from build123d import *

# Parameters (mm, degrees)
SKETCH1_R           = 6.5
BOSS_EXTRUDE1_DEPTH = 12
FILLET1_R           = 1


with BuildPart() as part:
    # Sketch1 → Boss-Extrude1 (new body)
    with BuildSketch(Plane.XY):
        with BuildLine():
            Line((-26, 9.287087811), (-26, 16.75))
            Line((-26, 16.75), (0, 16.75))
            Line((0, 16.75), (0, 20.75))
            Line((0, 20.75), (-30, 20.75))
            Line((-30, 20.75), (-30, 9.287087811))
            ThreePointArc((-30, 9.287087811), (-28, -9.5), (-26, 9.287087811))
        make_face()
        with Locations((-28, 0)):
            Circle(SKETCH1_R, mode=Mode.SUBTRACT)
    boss_extrude1 = extrude(amount=BOSS_EXTRUDE1_DEPTH)

    # Mirror1: Boss-Extrude1 across plane
    add(boss_extrude1.mirror(Plane(origin=(0, 0, 0), x_dir=(0, 0, 1), z_dir=(1, 0, 0))))

    # Fillet1
    fillet1_edges = [part.edges().sort_by_distance(p)[0] for p in [
        (-30, 9.287087811, 6),
        (-30, 20.75, 6),
        (-26, 16.75, 6),
        (-26, 9.287087811, 6),
        (26, 9.287087811, 6),
        (30, 9.287087811, 6),
        (30, 20.75, 6),
        (26, 16.75, 6),
    ]]
    fillet(fillet1_edges, radius=FILLET1_R)


solid = part.part
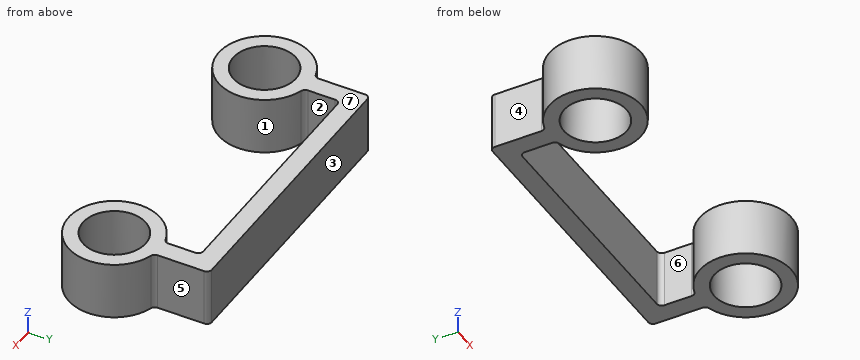
Can you work these out from the model? Positions are in its coordinate system, mm. Face numbers are marked on the shaded views. A direction names the side the tool comes from. Coordinates: 2 decimals unless noted, no trailing zeros. Order: outer loops, then holes, each group sorted by start corner. A loop starts at its lowest first (then second) coordinate and runs counter-clockwise, first axis right, second up. Notation, with made-up numbers: (33.5, -12.75) - (74.5, -12.75) arc R28 ccw to (74.5, 7.25) - close; hole circle Ø10 at (26.25, 41). An arc over 180 degrees is marked (long way). Answer as a JSON object with one key per item and string values. Group by question number.
Q1. Imagine slicing it at B-B (z = 1.5). Please give me the cut outline in (x, y), and give its area (3 significant figures).
Q2. On a 3-axis mill with a long thin cutter (end or side, diameter ignored), from which of +Z, -Z, +X, -X, +Y, -Y can I reach the whole of each face in a straight line? I mean the marked faces 5, 6 and 7. Say none if no direction works.
Q3. Imagine slicing it at A-A (x = -28). Please give me the cut outline in (y, z).
Q4. We'd pull the mould along X, two halves only. Please class the marked faces 1, 2, 3 and 4: +X half, -X half, draft (parallel to the pull), parting line (faces both ways), or undercut.
Q5. I need wall thicknesses on line 1 (Y direction, x = 28, z = 8); line 2 (X direction, y = 13, z = 5.25); line 3 (X direction, y = -4, z = 6). Which ranges of each line are inside material? Lowest first, please. Write a range as from..to.
Q6. Imagine slicing it at C-C (y = 0). Please give me the cut outline in (x, z).
Q7. Imagine slicing it at D-D (y = 19). Please give me the cut outline in (x, z).
Q8. Will these pins go through, and if not, where does the flat tip stop? P1, Ø3, axis at y = 11, z = 1.5, coming from the +X side; P2, Ø3, axis at y = 13, z = 6, coming from the +X side; P3, Ø10.5, axis at x = 28, y = 0, coming from the -Z side; P4, Ø1.7, axis at y = 12.5, z = 5, coming from the -X side.
Determined:
{
 "1": {"outline": "(-30.71, 9.1) arc R9.5 ccw (long way) to (-25.29, 9.1) arc R1 cw to (-26, 10.06) - (-26, 15.75) arc R1 cw to (-25, 16.75) - (25, 16.75) arc R1 cw to (26, 15.75) - (26, 10.06) arc R1 cw to (25.29, 9.1) arc R9.5 ccw (long way) to (30.71, 9.1) arc R1 cw to (30, 10.06) - (30, 19.75) arc R1 ccw to (29, 20.75) - (-29, 20.75) arc R1 ccw to (-30, 19.75) - (-30, 10.06) arc R1 cw to start; hole circle Ø13 at (-28, 0); hole circle Ø13 at (28, 0)", "area": "601 mm2"},
 "2": {"face 5": "+Z, -Z, +X, +Y", "face 6": "+Z, -Z", "face 7": "+Z, +X, -X, +Y, -Y"},
 "3": {"outline": "(-9.5, 0) - (-6.5, 0) - (-6.5, 12) - (-9.5, 12) - close; (6.5, 0) - (20.75, 0) - (20.75, 12) - (6.5, 12) - close"},
 "4": {"face 1": "undercut", "face 2": "undercut", "face 3": "draft", "face 4": "-X half"},
 "5": {"line 1": "y = -9.5..-6.5, 6.5..20.75", "line 2": "x = -30..-26, 26..30", "line 3": "x = -36.62..-33.12, -22.88..-19.38, 19.38..22.88, 33.12..36.62"},
 "6": {"outline": "(-37.5, 0) - (-34.5, 0) - (-34.5, 12) - (-37.5, 12) - close; (-21.5, 0) - (-18.5, 0) - (-18.5, 12) - (-21.5, 12) - close; (18.5, 0) - (21.5, 0) - (21.5, 12) - (18.5, 12) - close; (34.5, 0) - (37.5, 0) - (37.5, 12) - (34.5, 12) - close"},
 "7": {"outline": "(-30, 0) - (30, 0) - (30, 12) - (-30, 12) - close"},
 "8": {"P1": "stops at x = 30.17", "P2": "stops at x = 30", "P3": "passes through", "P4": "stops at x = -30"}
}
